```python
from build123d import *

# Parameters (mm, degrees)
BOSS_EXTRUDE1_DEPTH = 12.7
SKETCH3_R           = 3.937
CUT_EXTRUDE1_DEPTH  = 539.366167213
SKETCH4_R           = 1.524
SKETCH4_R_2         = 3.937
CUT_EXTRUDE2_DEPTH  = 539.366167213


with BuildPart() as part:
    # Sketch2 → Boss-Extrude1 (new body)
    with BuildSketch(Plane.XY):
        with BuildLine():
            Line((0, 0), (431.8, 0))
            ThreePointArc((431.8, 0), (485.681536726, 22.318463274), (508, 76.2))
            Line((508, 76.2), (508, 101.6))
            ThreePointArc((508, 101.6), (485.681536726, 155.481536726), (431.8, 177.8))
            Line((431.8, 177.8), (152.4, 177.8))
            Line((152.4, 177.8), (76.2, 177.8))
            Line((76.2, 177.8), (76.2, 61.401251199))
            ThreePointArc((76.2, 61.401251199), (33.506060073, 36.401783403), (0, 0))
        make_face()
    extrude(amount=BOSS_EXTRUDE1_DEPTH)

    # Sketch3 → Cut-Extrude1 (cut, through all)
    with BuildSketch(Plane(origin=(0, 0, 0), x_dir=(-1, 0, 0), z_dir=(0, 0, -1))):
        with Locations((-177.8, 29.082055279)):
            Circle(SKETCH3_R)
        with Locations((-400.836394982, 29.082055279)):
            Circle(SKETCH3_R)
        with Locations((-400.836394982, 151.002055279)):
            Circle(SKETCH3_R)
        with Locations((-177.8, 151.002055279)):
            Circle(SKETCH3_R)
    extrude(amount=-CUT_EXTRUDE1_DEPTH, mode=Mode.SUBTRACT)

    # Sketch4 → Cut-Extrude2 (cut, through all)
    with BuildSketch(Plane.XY.offset(12.7)):
        with Locations((292.1, 76.2)):
            Circle(SKETCH4_R)
        with Locations((237.998, 76.2)):
            Circle(SKETCH4_R_2)
        with Locations((346.202, 76.2)):
            Circle(SKETCH4_R_2)
    extrude(amount=-CUT_EXTRUDE2_DEPTH, mode=Mode.SUBTRACT)


solid = part.part
```
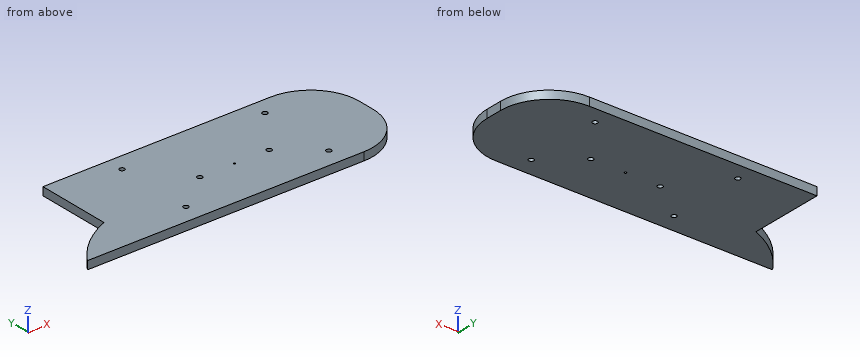
Verification items for the finished model (mm, model axes). Round coordinates to 2 decimals unless told otherwise and drop trailing zeros. Write each loop counter-clockwise with the first axis right and the second up, starting at its lowest first coordinate (ties: lowest second). Pieces come first, ordered by that corner, then holes.
1. Scan lines: L1, parallel to Y at x = 177.8, z = 8.75; L2, parallel to X at y = 78, z = 1; L3, parallel to X at y = 26, z = 7.75. Record each from-to range of solid material in increasing order.
2. Section check C-C on y = 117. Enter the section's corners in (x, z), plus the area to 3 significant figures.
3. Section check A-A on z = 2.5. Enter the section's corners in (x, y) (3 decimals).
4. Section check B-B on y = 87. Enter the section's corners in (x, z), plus the area to 3 significant figures.
5. Gauge pin test, flat ends, axial feed: P1, Ø1.5, axis at y = 19, z = 11.5, coming from the -X side; P2, Ø3, axis at y = 154, z = 3, coming from the -X side. Record the tip position at first contact, or that the pin passes through.
Answer:
1. L1: y = 0 to 25.15, 33.02 to 147.07, 154.94 to 177.8
1. L2: x = 76.2 to 234.5, 241.5 to 342.7, 349.7 to 508
1. L3: x = 21.77 to 175.35, 180.25 to 398.39, 403.29 to 489.13
2. outline: (76.2, 0) - (506.43, 0) - (506.43, 12.7) - (76.2, 12.7) - close
2. area: 5,460 mm2
3. outline: (0, 0) - (431.8, 0) arc R76.2 ccw to (508, 76.2) - (508, 101.6) arc R76.2 ccw to (431.8, 177.8) - (76.2, 177.8) - (76.2, 61.401) arc R167.157 ccw to start; hole circle Ø7.874 at (177.8, 29.082); hole circle Ø7.874 at (177.8, 151.002); hole circle Ø7.874 at (237.998, 76.2); hole circle Ø3.048 at (292.1, 76.2); hole circle Ø7.874 at (346.202, 76.2); hole circle Ø7.874 at (400.836, 29.082); hole circle Ø7.874 at (400.836, 151.002)
4. outline: (76.2, 0) - (508, 0) - (508, 12.7) - (76.2, 12.7) - close
4. area: 5,480 mm2
5. P1: stops at x = 14.31
5. P2: stops at x = 76.2
